Source: three-view drawing plus pictorial views. Frame: mm from the lowest corner of the part. Give positions to 0.01 mm unless a question says otherwise; leave off trailing zeros. Loops run counter-clockwise (first coordinate to the right, second up) from the corner with the lowest first, then second, coordinate; pieces in that order, holes last. Notation, with made-up numbers: (-30.75, 29.25) - (-10.75, 29.25) arc R23 cw to (-10.75, 39.25) - close; hole circle Ø4 at (37, -35). An arc over 180 degrees is marked (long way). Write each question's results on one line, items separated by ' | '. Start each with the question number.
(1) Contact query for flat-ended pins moving along their axis: pin 1 (8 mm diameter, centred on x = 100, z = 9, fed in from +Y); pin 2 (1 mm diameter, centred on y = 17, z = 6, fed in from +X). Output: stop coordinate, or through.
(2) Pull-direction query (Y, two-part tool) for the marked faces 1, 2 and 3; classes: pulls with the +Y half, pulls with the -Y half, needs draft (parallel to the pull), parting line crosses it, or undercut.
(3) Material intervals for line 1 along X through (y, z) = (4, 9); line 2 along Y through (x, z) = (33, 8.25); line 3 along X through (y, z) = (8.75, 2), sorted ascending. Write a range as [from, to].
(4) Cut plane B-B on x = 33. Return the cut outline in (y, z).
(5) Cut plane A-A on z = 9. Return the cut outline in (x, y), then the cut area to 3 significant figures.
(6) Cut plane D-D on y = 2.25. Return the cut outline in (x, z), then the cut area to 3 significant figures.
(7) Cut plane C-C on y = 10.5. Return the cut outline in (x, z).
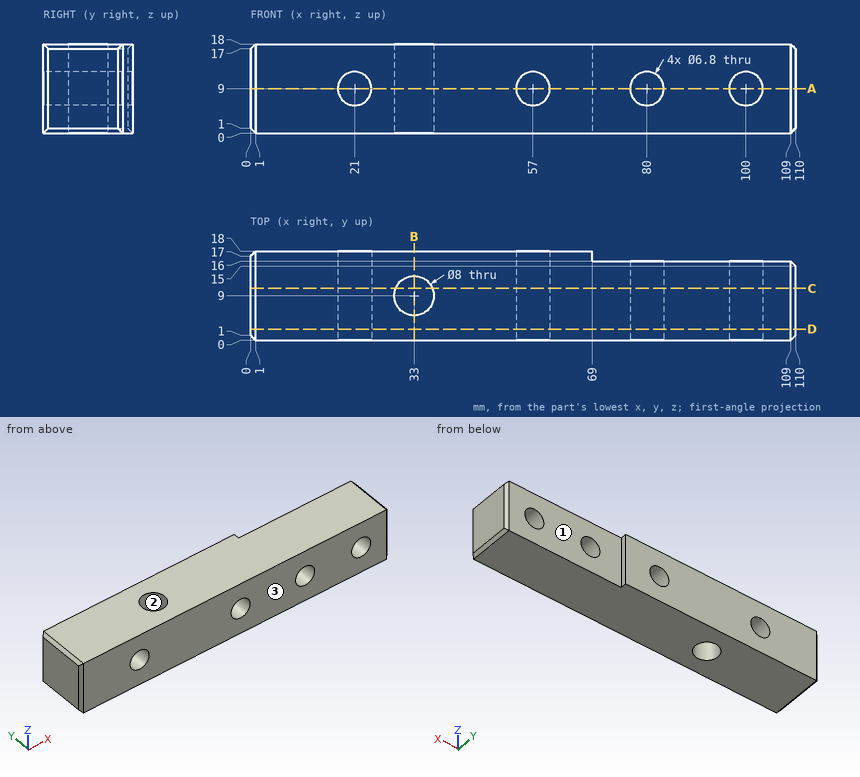
Ans:
1) pin 1: y = 16 | pin 2: x = 69
2) face 1: pulls with the +Y half | face 2: undercut | face 3: pulls with the -Y half
3) line 1: [0, 17.6], [24.4, 53.6], [60.4, 76.6], [83.4, 96.6], [103.4, 110] | line 2: [0, 5], [13, 18] | line 3: [0, 29.01], [36.99, 110]
4) outline: (0, 0) - (5, 0) - (5, 18) - (0, 18) - close; (13, 0) - (18, 0) - (18, 18) - (13, 18) - close
5) outline: (0, 1) - (1, 0) - (17.6, 0) - (17.6, 18) - (1, 18) - (0, 17) - close; (24.4, 0) - (53.6, 0) - (53.6, 18) - (24.4, 18) - close; (60.4, 0) - (76.6, 0) - (76.6, 16) - (69, 16) - (69, 18) - (60.4, 18) - close; (83.4, 0) - (96.6, 0) - (96.6, 16) - (83.4, 16) - close; (103.4, 0) - (109, 0) - (110, 1) - (110, 15) - (109, 16) - (103.4, 16) - close; hole circle Ø8 at (33, 9) | area: 1,380 mm^2
6) outline: (0, 1) - (1, 0) - (109, 0) - (110, 1) - (110, 17) - (109, 18) - (1, 18) - (0, 17) - close; hole circle Ø6.8 at (21, 9); hole circle Ø6.8 at (57, 9); hole circle Ø6.8 at (80, 9); hole circle Ø6.8 at (100, 9) | area: 1,830 mm^2
7) outline: (0, 1) - (1, 0) - (29.29, 0) - (29.29, 18) - (1, 18) - (0, 17) - close; (36.71, 0) - (109, 0) - (110, 1) - (110, 17) - (109, 18) - (36.71, 18) - close; hole circle Ø6.8 at (21, 9); hole circle Ø6.8 at (57, 9); hole circle Ø6.8 at (80, 9); hole circle Ø6.8 at (100, 9)
